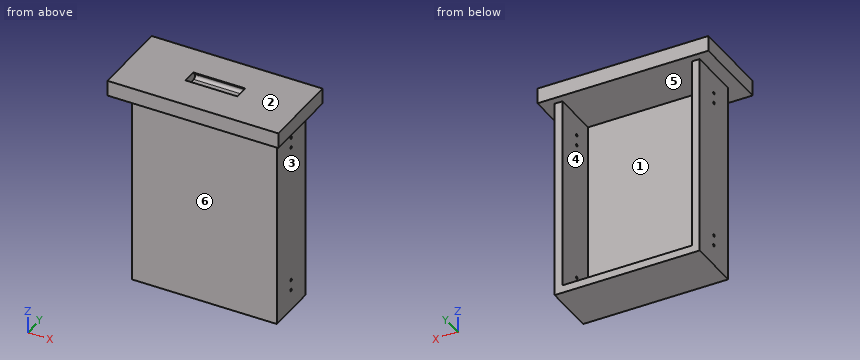
```python
from build123d import *

# Parameters (mm, degrees)
SKETCH1_W           = 330
SKETCH1_H           = 155
BOSS_EXTRUDE1_DEPTH = 30
SKETCH2_W           = 280
SKETCH2_H           = 100
BOSS_EXTRUDE2_DEPTH = 390
SKETCH3_W           = 250
SKETCH3_H           = 375
CUT_EXTRUDE1_DEPTH  = 90
CUT_EXTRUDE2_DEPTH  = 50
FILLET1_R           = 0.5
SKETCH7_R           = 2.5
CUT_EXTRUDE3_DEPTH  = 502.129973161


with BuildPart() as part:
    # Sketch1 → Boss-Extrude1 (new body)
    with BuildSketch(Plane.XY):
        Rectangle(SKETCH1_W, SKETCH1_H)
    extrude(amount=BOSS_EXTRUDE1_DEPTH)

    # Sketch2 → Boss-Extrude2 (add)
    with BuildSketch(Plane(origin=(0, 0, 0), x_dir=(-1, 0, 0), z_dir=(0, 0, -1))):
        with Locations((0, 12.5)):
            Rectangle(SKETCH2_W, SKETCH2_H)
    extrude(amount=BOSS_EXTRUDE2_DEPTH)

    # Sketch3 → Cut-Extrude1 (cut)
    with BuildSketch(Plane(origin=(0, 62.5, 0), x_dir=(1, 0, 0), z_dir=(0, 1, 0))):
        with Locations((0, 187.5)):
            Rectangle(SKETCH3_W, SKETCH3_H)
    extrude(amount=-CUT_EXTRUDE1_DEPTH, mode=Mode.SUBTRACT)

    # Sketch4 → Cut-Extrude2 (cut, symmetric)
    with BuildSketch(Plane(origin=(0, 0, 0), x_dir=(0, 0, -1), z_dir=(1, 0, 0))):
        with BuildLine():
            Line((-35.714873599, 8.791050276), (-23.35130712, 19.957391338))
            ThreePointArc((-23.35130712, 19.957391338), (-17.969795035, 20.816040293), (-15, 16.246765975))
            Line((-15, 16.246765975), (-15, -2.5))
            ThreePointArc((-15, -2.5), (-33.319001977, -11.460982872), (-35.714873599, 8.791050276))
        make_face()
    extrude(amount=CUT_EXTRUDE2_DEPTH, both=True, mode=Mode.SUBTRACT)

    # Fillet1
    fillet1_edges = [part.edges().sort_by_distance(p)[0] for p in [
        (0, 13.952524341, 30),
    ]]
    fillet(fillet1_edges, radius=FILLET1_R)

    # Sketch7 → Cut-Extrude3 (cut, through all)
    with BuildSketch(Plane(origin=(140, 0, 0), x_dir=(0, 0, -1), z_dir=(1, 0, 0))):
        with Locations((350, 12.5)):
            Circle(SKETCH7_R)
        with Locations((330, 12.5)):
            Circle(SKETCH7_R)
        with Locations((60, 12.5)):
            Circle(SKETCH7_R)
        with Locations((40, 12.5)):
            Circle(SKETCH7_R)
    extrude(amount=-CUT_EXTRUDE3_DEPTH, mode=Mode.SUBTRACT)


solid = part.part
```
Geometry check sheet. Reference: the model listing, model coordinates, mm. Face numbers are marked on the shaded views. A direction names the side the tool comes from. Round coordinates to 2 decimals unless told otherwise and drop trailing zeros. Loops run counter-clockwise (first coordinate to the right, second up) from the corner with the lowest first, then second, coordinate; pieces in that order, holes last. Notation, with made-up numbers: (53, 28.5) -> (69, 28.5) arc R14 ccw to (69, 34.5) -> close; hole circle Ø1 at (31, -0.75). An arc over 180 degrees is marked (long way). Use a Markdown table: item, result.
(1) Sectioned sample at C-C (y = 67.5). Enter the section's corners in (x, z).
Calculated:
| item | result |
|---|---|
| outline | (-165, 0) -> (165, 0) -> (165, 30) -> (-165, 30) -> close |
(2) Set-up check for the marked faces 4, 5 and 6: record each of +Z, -Z, +X, -X, +Y, -Y from which the full face is reachable in a straight line by a thin tool's end or side.
Calculated:
| item | result |
|---|---|
| face 4 | +Y |
| face 5 | none |
| face 6 | -Z, +X, -X, -Y |
(3) Go/stop test with flat-tipped pins: P1, Ø1.5, axis at x = -98, y = -49, coming from the -Z side; P2, Ø4, axis at y = -32.5, z = -122, coming from the -X side; P3, Ø12, axis at y = 36, z = -101, coming from the +X side. Record where each tip stops, or that it passes through.
Calculated:
| item | result |
|---|---|
| P1 | z = 0 |
| P2 | x = -140 |
| P3 | x = 140 |
(4) Sectioned sample at D-D (x = -2). Enter the section's corners in (y, z).
Calculated:
| item | result |
|---|---|
| outline | (-77.5, 0) -> (-37.5, 0) -> (-37.5, -390) -> (62.5, -390) -> (62.5, -375) -> (-27.5, -375) -> (-27.5, 0) -> (77.5, 0) -> (77.5, 30) -> (15.08, 30) arc R0.5 ccw to (14.71, 29.16) -> (19.96, 23.35) arc R5 cw to (16.25, 15) -> (-2.5, 15) arc R12.5 cw to (-12.7, 30) -> (-77.5, 30) -> close |
(5) Mould release check, pull along Z, two halves, no side actions. Record for the marked faces 1, 2 and 3: released by +Z, released by -Z, zero draft, split by the parting line, or undercut.
Calculated:
| item | result |
|---|---|
| face 1 | undercut |
| face 2 | released by +Z |
| face 3 | zero draft |
(6) Sectioned sample at B-B (z = -316). Enter the section's corners in (x, y), then the cut area to 3 significant figures.
Calculated:
| item | result |
|---|---|
| outline | (-140, -37.5) -> (140, -37.5) -> (140, 62.5) -> (125, 62.5) -> (125, -27.5) -> (-125, -27.5) -> (-125, 62.5) -> (-140, 62.5) -> close |
| area | 5,500 mm² |
(7) Scan lines: probe 1 along Z at (x, y) = (-80.5, 58.5); probe 2 along Y at (x, z) = (-129, -350); probe 3 along X at (y, z) = (23, -187.5). Record each from-to range of solid material in increasing order.
Calculated:
| item | result |
|---|---|
| probe 1 | -390 to -375, 0 to 30 |
| probe 2 | -37.5 to 10, 15 to 62.5 |
| probe 3 | -140 to -125, 125 to 140 |
(8) Sectioned sample at A-A (x = 59). Enter the section's corners in (y, z).
Calculated:
| item | result |
|---|---|
| outline | (-77.5, 0) -> (-37.5, 0) -> (-37.5, -390) -> (62.5, -390) -> (62.5, -375) -> (-27.5, -375) -> (-27.5, 0) -> (77.5, 0) -> (77.5, 30) -> (-77.5, 30) -> close |
